Check sheet for the modelled part. Datum: model origin and axes. Units: mm. Coordinates: 2 decimals unless noted, no trailing zeros. Loops run counter-clockwise (first coordinate to the right, second up) from the corner with the lowest first, then second, coordinate; pieces in that order, holes last. Notation, with made-up numbers: M 58.25,15 L 110.25,15 A23 cw 110.25,25 Z; hole C 61.25,44.25 d11. An arc over 180 degrees is marked long. Answer as CSV lines item,"result". Start each with the question number.
Autodesk Inventor part; units mm, degrees
ref_plane "YZ Plane" through (0, 0, 0) normal (1, 0, 0) x (0, 1, 0)
ref_plane "XZ Plane" through (0, 0, 0) normal (0, 1, 0) x (-1, 0, 0)
ref_plane "XY Plane" through (0, 0, 0) normal (0, 0, 1) x (1, 0, 0)
sketch "Sketch1" plane through (0, 0, 0) normal (0, 0, 1) x (1, 0, 0)
  line L0 (0, 0) -> (-154.6388, 0)
  line L1 (-154.6388, 0) -> (-154.6388, -1500)
  line L2 (-154.6388, -1500) -> (0, -1500)
  line L3 (0, -1500) -> (0, 0)
  line L4 (-154.6388, -1400) -> (-81, -1400)
  line L5 (-81, -1400) -> (-81, -1394)
  line L6 (-81, -1394) -> (-154.6388, -1394)
  line L7 (-154.6388, -1394) -> (-154.6388, -1400)
  line L8 (-154.6388, -900) -> (-81, -900)
  line L9 (-81, -900) -> (-81, -894)
  line L10 (-81, -894) -> (-154.6388, -894)
  line L11 (-154.6388, -894) -> (-154.6388, -900)
  line L12 (-154.6388, -400) -> (-81, -400)
  line L13 (-81, -400) -> (-81, -394)
  line L14 (-81, -394) -> (-154.6388, -394)
  line L15 (-154.6388, -394) -> (-154.6388, -400)
  point P0 (-154.6388, -900)
  point P1 (-154.6388, -1394)
  dimension "d0" = 1500
  dimension "d1" = 154.6388
  dimension "d2" = 6
  dimension "d4" = 100
  dimension "d7" = 500
  dimension "d23" = 81
extrude "Plate1" add sketch "Sketch1" along normal blind 4 contours L3 L2 L1 L4 L5 L6 L8 L9 L10 L12 L13 L14 L0
sketch "Sketch2" plane through (4, 0, 0) normal (-1, 0, 0) x (0, -1, 0)
  line L0 (1500, 0) -> (0, 0)
  line L1 (0, 0) -> (0, 35)
  line L2 (0, 35) -> (1500, 35)
  line L3 (1500, 35) -> (1500, 0)
edge flange "Flange1" height 35 angle 90 thickness 4 bend radius 4 thickness toward (-1, 0, 0) relief tear relief width 4 relief depth 2 edges at (0, -750, 4) wall of the first edge with corners at (4, -1500, 0) (4, 0, 0) (4, 0, 35) (4, -1500, 35)
bend "Bend1"
corner "Corner1"
equation "\"d1\" = Stringer2_2_deep"
equation "\"d12\" = Thickness"
equation "\"d13\" = BendReliefWidth"
equation "\"d14\" = BendReliefDepth"
equation "\"d15\" = MinimumRemnant"
equation "\"d16\" = TransitionRadius"
equation "\"d19\" = BendRadius"
equation "\"d20\" = CornerReliefSize"
equation "\"d21\" = GapSize"
equation "\"d22\" = JacobiRadiusSize"
equation "\"BendRadius\" = Thickness"
equation "\"BendReliefWidth\" = Thickness"
equation "\"BendReliefDepth\" = 0.5 * Thickness"
equation "\"CornerReliefSize\" = 4 * Thickness"
equation "\"MinimumRemnant\" = 2 * Thickness"
equation "\"TransitionRadius\" = BendRadius"
equation "\"JacobiRadiusSize\" = BendRadius"
equation "\"GapSize\" = Thickness"
properties part number "stringer 1.2_CPY2"
Item 1: Sectioned sample at A-A, the plane x = -98. Record the boundary of the cut face in (y, z), and give its area (3 significant figures).
Item 2: Go/stop test with flat-tipped pins: pin 1 (1.2 mm diameter, centred on x = -111, z = 2, fed in from +Y); pin 2 (1.5 mm diameter, centred on x = -55, y = -540.5, fed in from +Z); pin 3 (4.5 mm diameter, centred on y = -396.5, z = 3, fed in from -X); pin 4 (8 mm diameter, centred on y = -666.5, z = 23.5, fed in from -X). Record where each tip stops, or that it passes through.
Item 3: Sectioned sample at C-C, the plane z = 18. Record the boundary of the cut face in (x, y), and give its area (3 significant figures).
Item 4: Release check for a two-part mould opening along X. For faces 1 (the face through (-80, -740, 4)), 2 (the face through (0, -740, 21)), 3 (the face through (4, -740, 22)) record: released by +X, released by -X, zero draft, split by the parting line, or undercut.
Item 5: Sectioned sample at B-B, the plane y = -686.5. Record the boundary of the cut face in (x, z), and give its area (3 significant figures).
Item 6: Material ranges on line 1 (X direction, y = -707, z = 32); line 2 (X direction, y = -489.5, z = 3) (3 decimals), recorded low to high. Write a range as from..to.
Reply:
1,outline,"M -1500,0 L -1400,0 L -1400,4 L -1500,4 Z; M -1394,0 L -900,0 L -900,4 L -1394,4 Z; M -894,0 L -400,0 L -400,4 L -894,4 Z; M -394,0 L 0,0 L 0,4 L -394,4 Z"
1,area,"5,930 mm²"
2,pin 1,"y = 0"
2,pin 2,"z = 4"
2,pin 3,"x = -81"
2,pin 4,"x = 0"
3,outline,"M 0,-1500 L 4,-1500 L 4,0 L 0,0 Z"
3,area,"6,000 mm²"
4,face 1,"zero draft"
4,face 2,"released by -X"
4,face 3,"released by +X"
5,outline,"M -154.64,0 L -4,0 A8 ccw 4,8 L 4,35 L 0,35 L 0,8 A4 cw -4,4 L -154.64,4 Z"
5,area,"748 mm²"
6,line 1,"0..4"
6,line 2,"-154.639..2.245"
